from build123d import *

# Parameters (mm, degrees)
PERFORADOR_PARA_ROSCAR_PARA_MACHO_DE_ROS_D     = 4.2
PERFORADOR_PARA_ROSCAR_PARA_MACHO_DE_ROS_DEPTH = 20
PERFORADOR_PARA_ROSCAR_PARA_MACHO_DE_ROS_TIP   = 1.2618073
PERFORADOR_PARA_ROSCAR_PARA_MACHO_DE_2_D       = 4.2
PERFORADOR_PARA_ROSCAR_PARA_MACHO_DE_2_DEPTH   = 20
PERFORADOR_PARA_ROSCAR_PARA_MACHO_DE_2_TIP     = 1.2618073
PERFORADOR_PARA_ROSCAR_PARA_MACHO_DE_3_D       = 8.5
PERFORADOR_PARA_ROSCAR_PARA_MACHO_DE_3_DEPTH   = 40
PERFORADOR_PARA_ROSCAR_PARA_MACHO_DE_3_TIP     = 2.553657631


with BuildPart() as part:
    # Croquis1 → Revolución1 (revolve)
    with BuildSketch(Plane.XY, mode=Mode.PRIVATE) as revoluci_n1_sk:
        Polygon((16.35, 24.5), (20, 24.5), (20, 20), (35, 20), (35, 0), (0, 0), (0, 24.5), (3.65, 24.5), (8.232717762, 16.5625), (11.767282238, 16.5625), align=None)
    revolve(revoluci_n1_sk.sketch.rotate(Axis((0, 0, 0), (1, 0, 0)), 90), axis=Axis((0, 0, 0), (1, 0, 0)))

    # Perforador para roscar para macho de ros
    with Locations(Plane(origin=(28, 0, 20), x_dir=(1, 0, 0), z_dir=(0, 0, 1))):
        with Locations((0, 0)):
            Hole(PERFORADOR_PARA_ROSCAR_PARA_MACHO_DE_ROS_D / 2, depth=PERFORADOR_PARA_ROSCAR_PARA_MACHO_DE_ROS_DEPTH)
            with Locations((0, 0, -(PERFORADOR_PARA_ROSCAR_PARA_MACHO_DE_ROS_DEPTH + PERFORADOR_PARA_ROSCAR_PARA_MACHO_DE_ROS_TIP / 2))):  # 118° drill point
                Cone(0, PERFORADOR_PARA_ROSCAR_PARA_MACHO_DE_ROS_D / 2, PERFORADOR_PARA_ROSCAR_PARA_MACHO_DE_ROS_TIP, mode=Mode.SUBTRACT)

    # Perforador para roscar para macho de 2
    with Locations(Plane(origin=(28, 19.999069745, -0.192897185), x_dir=(0, 0.009645004686, 0.999953485861), z_dir=(0, 0.999953485861, -0.009645004686))):
        with Locations((0, 0)):
            Hole(PERFORADOR_PARA_ROSCAR_PARA_MACHO_DE_2_D / 2, depth=PERFORADOR_PARA_ROSCAR_PARA_MACHO_DE_2_DEPTH)
            with Locations((0, 0, -(PERFORADOR_PARA_ROSCAR_PARA_MACHO_DE_2_DEPTH + PERFORADOR_PARA_ROSCAR_PARA_MACHO_DE_2_TIP / 2))):  # 118° drill point
                Cone(0, PERFORADOR_PARA_ROSCAR_PARA_MACHO_DE_2_D / 2, PERFORADOR_PARA_ROSCAR_PARA_MACHO_DE_2_TIP, mode=Mode.SUBTRACT)

    # Perforador para roscar para macho de 3
    with Locations(Plane(origin=(35, 0, 0), x_dir=(0, 0, -1), z_dir=(1, 0, 0))):
        with Locations((0, 0)):
            Hole(PERFORADOR_PARA_ROSCAR_PARA_MACHO_DE_3_D / 2, depth=PERFORADOR_PARA_ROSCAR_PARA_MACHO_DE_3_DEPTH)
            with Locations((0, 0, -(PERFORADOR_PARA_ROSCAR_PARA_MACHO_DE_3_DEPTH + PERFORADOR_PARA_ROSCAR_PARA_MACHO_DE_3_TIP / 2))):  # 118° drill point
                Cone(0, PERFORADOR_PARA_ROSCAR_PARA_MACHO_DE_3_D / 2, PERFORADOR_PARA_ROSCAR_PARA_MACHO_DE_3_TIP, mode=Mode.SUBTRACT)


solid = part.part
Source: CAD feature listing. Evaluate the final solid. Frame: model axes, mm. A direction names the side the tool comes from. Round coordinates to 2 decimals unless told otherwise and drop trailing zeros. Write each loop counter-clockwise with the first axis right and the second up, starting at its lowest first coordinate (ties: lowest second). Pieces come first, ordered by that corner, then holes. Notation, with made-up numbers: M 32.25,19 L 91.25,19 A27 ccw 91.25,50 Z; hole C 26.5,47.25 d3. An arc over 180 degrees is marked long. One line per item, written item: value. Start each with the question number.
Item 1: Set-up query: faces 4 (the cylindrical face through (18.2, -7.36, 23.37)), 5 (the flat face through (20, 18, -9.2)), 6 (the cylindrical face through (26.137, 11.725, -1.082)). Return all of +Z, -Z, +X, -X, +Y, -Y with unobstructed straight access to the full face (end or side cutting, diameter ignored); none if empty.
Item 2: Section query C-C (z = 18). State how many separate pieces and enclosed holes the cut face has, plus the area to 3 significant figures.
Item 3: Ray query, L1, parallel to X at y = 0, z = 11; L2, parallel to X at y = 19, z = 6; L3, parallel to Z at x = 4, y = -1.5. Return the intervals inside material, ascending. Write a range as from..to.
Item 4: Mould query, pull axis Y, two halves, no side actions, for faces 1 (the cylindrical face through (30.1, 0.09, 11.73)), 2 (the conical face through (12.054, -5.124, 16.271)), 3 (the flat face through (35, -5, 0)). Classes: pulls with the +Y half, pulls with the -Y half, needs draft (parallel to the pull), parting line crosses it, or undercut.
Item 5: Section query A-A (y = 0). Return the cut outline in (x, z), plus the area to 3 significant figures.
Item 6: Pin query (flat end, axial travel): pin 1 (12 mm diameter, centred on x = 20, z = -8.5, fed in from +Y); pin 2 (1.5 mm diameter, centred on x = 13, z = 3, fed in from -Y); pin 3 (1 mm diameter, centred on x = 11.5, y = 4, fed in from -Z). Return the tip coordinate at first contact, or that it passes through.
Result set:
1. face 4: +X, -X
1. face 5: +X
1. face 6: none
2. separate pieces: 2
2. enclosed holes: 1
2. area: 651 mm²
3. L1: x = 0..25.9, 30.1..35
3. L2: x = 0..6.29, 13.71..35
3. L3: z = -23.85..-3.98, 3.98..23.85
4. face 1: undercut
4. face 2: parting line crosses it
4. face 3: needs draft
5. outline: M 0,-24.5 L 3.65,-24.5 L 8.23,-16.56 L 11.77,-16.56 L 16.35,-24.5 L 20,-24.5 L 20,-20 L 35,-20 L 35,-4.25 L 0,-4.25 Z; M 0,4.25 L 25.9,4.25 L 25.9,20 L 20,20 L 20,24.5 L 16.35,24.5 L 11.77,16.56 L 8.23,16.56 L 3.65,24.5 L 0,24.5 Z; M 30.1,4.25 L 35,4.25 L 35,20 L 30.1,20 Z
5. area: 1,090 mm²
6. pin 1: stops at y = 24.37
6. pin 2: stops at y = -19.78
6. pin 3: stops at z = -16.5
